Here's the drawing with two shaded views (mm, measured from the low corner). I have some questions. A direction names the side the tool comes from. Give positions to 0.01 mm unless a question says otherwise; leave off trailing zeros. Order: outer loops, then holes, each group sorted by start corner. A loop starts at its lowest first (then second) coordinate and runs counter-clockwise, first axis right, second up. Notation, with made-up numbers: M 78,-14 L 106,-14 A14 ccw 106,-2 Z; hole C 81.25,41.25 d11. An arc over 180 degrees is marked long. Use a Markdown table: item, result. Add a question column.
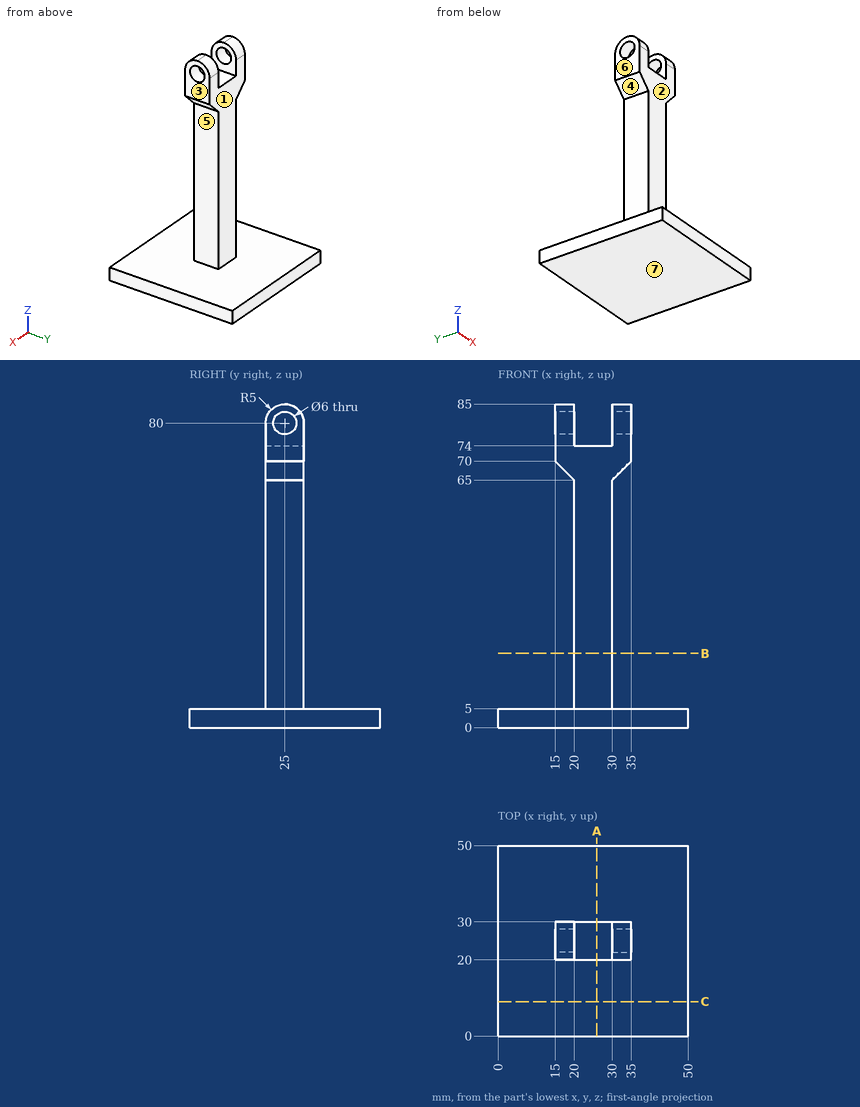
1. We'd pull the mould along Z, two halves only. Please class the marked faces 5, 6 and 7: +Z half, -Z half, draft (parallel to the pull), parting line (faces both ways), or undercut.
2. On a 3-axis mill with a long thin cutter (end or side, diameter ignored), from which of +Z, -Z, +X, -X, +Y, -Y can I reach the whole of each face in a straight line? I mean the marked faces 1, 2, 3 and 4. Say none if no direction works.
3. I need wall thicknesses on L1, parallel to Z at x = 33, y = 25; L2, parallel to Z at x = 32.4, y = 25; L3, parallel to Z at x = 15, y = 37. Which ranges of each line are inside material? Lowest first, please. Write a range as [from, to].
4. If we section it at C-C, the plane y = 9: List the corners of the cut face in (x, z) for me.
5. If we section it at B-B, the plane z = 19.5: List the corners of the cut face in (x, y) for me, then the cut area to 3 significant figures.
6. Will these pins go through, and if not, where does the flat tip stop? pin 1 (3 mm diameter, centred on x = 38.5, y = 12, fed in from +Z); pin 2 (10 mm diameter, centred on x = 24, z = 49.5, fed in from +Y); pin 3 (11 mm diameter, centred on y = 22.5, z = 76.5, fed in from -X).
7. If we section it at A-A, the plane x = 26: List the corners of the cut face in (y, z) for me.
Geometry results:
| question | item | result |
|---|---|---|
| 1 | face 5 | undercut |
| 1 | face 6 | draft |
| 1 | face 7 | -Z half |
| 2 | face 1 | +Z, +X, -X, +Y |
| 2 | face 2 | +Z, +X, -X, -Y |
| 2 | face 3 | +Z, +X, +Y, -Y |
| 2 | face 4 | -X, +Y, -Y |
| 3 | L1 | z = [0, 5], [68, 77], [83, 85] |
| 3 | L2 | z = [0, 5], [67.4, 77], [83, 85] |
| 3 | L3 | z = [0, 5] |
| 4 | outline | M 0,0 L 50,0 L 50,5 L 0,5 Z |
| 5 | outline | M 20,20 L 30,20 L 30,30 L 20,30 Z |
| 5 | area | 100 mm^2 |
| 6 | pin 1 | stops at z = 5 |
| 6 | pin 2 | stops at y = 30 |
| 6 | pin 3 | stops at x = 15 |
| 7 | outline | M 0,0 L 50,0 L 50,5 L 30,5 L 30,74 L 20,74 L 20,5 L 0,5 Z |
